from build123d import *

# Parameters (mm, degrees)
SKETCH1_R           = 22.86
BOSS_EXTRUDE1_DEPTH = 22.86
SKETCH3_R           = 15.24
BOSS_EXTRUDE2_DEPTH = 55.88
SKETCH4_R           = 22.86
BOSS_EXTRUDE3_DEPTH = 22.86
FILLET3_R           = 2.54
SKETCH5_R           = 2.055
CUT_EXTRUDE1_DEPTH  = 7.62
SKETCH8_W           = 3.7
SKETCH8_H           = 3.4
CUT_EXTRUDE2_DEPTH  = 85
FILLET4_R           = 1


with BuildPart() as part:
    # Sketch1 → Boss-Extrude1 (new body)
    with BuildSketch(Plane(origin=(0, 0, 0), x_dir=(1, 0, 0), z_dir=(0, 1, 0))):
        Circle(SKETCH1_R)
    extrude(amount=BOSS_EXTRUDE1_DEPTH)

    # Sketch3 → Boss-Extrude2 (add)
    with BuildSketch(Plane(origin=(0, 22.86, 0), x_dir=(1, 0, 0), z_dir=(0, 1, 0))):
        Circle(SKETCH3_R)
    extrude(amount=BOSS_EXTRUDE2_DEPTH)

    # Sketch4 → Boss-Extrude3 (add)
    with BuildSketch(Plane(origin=(0, 78.74, 0), x_dir=(1, 0, 0), z_dir=(0, 1, 0))):
        Circle(SKETCH4_R)
    extrude(amount=BOSS_EXTRUDE3_DEPTH)

    # Fillet3
    fillet3_edges = [part.edges().sort_by_distance(p)[0] for p in [
        (-22.86, 101.6, 0),
        (-22.86, 0, 0),
    ]]
    fillet(fillet3_edges, radius=FILLET3_R)

    # Sketch5 → Cut-Extrude1 (cut)
    with BuildSketch(Plane(origin=(0, 101.6, 0), x_dir=(1, 0, 0), z_dir=(0, 1, 0))):
        Circle(SKETCH5_R)
    extrude(amount=-CUT_EXTRUDE1_DEPTH, mode=Mode.SUBTRACT)

    # Sketch8 → Cut-Extrude2 (cut)
    with BuildSketch(Plane.XZ):
        Rectangle(SKETCH8_W, SKETCH8_H)
    extrude(amount=-CUT_EXTRUDE2_DEPTH, mode=Mode.SUBTRACT)

    # Fillet4
    fillet4_edges = [part.edges().sort_by_distance(p)[0] for p in [
        (-2.055, 101.6, 0),
        (-1.85, 0, 0),
        (0, 0, -1.7),
        (1.85, 0, 0),
        (0, 0, 1.7),
    ]]
    fillet(fillet4_edges, radius=FILLET4_R)


solid = part.part
Build history of the part. All positions in model axes, mm. A direction names the side the tool comes from. Round coordinates to 2 decimals unless told otherwise and drop trailing zeros. Write each loop counter-clockwise with the first axis right and the second up, starting at its lowest first coordinate (ties: lowest second). Pieces come first, ordered by that corner, then holes. Notation, with made-up numbers: M -37.75,-35.5 L -4.75,-35.5 A20 ccw -4.75,1.5 Z; hole C 30,73.5 d4. An arc over 180 degrees is marked long. Use CSV: the item, a comma, the result in double quotes.
1. Saw through at C-C (z = 0). Give the cut face in (x, y) (3 decimals), plus the area to 3 significant figures.
Reply:
outline,"M -22.86,2.54 A2.54 ccw -20.32,0 L -2.85,0 A1 ccw -1.85,1 L -1.85,85 L 1.85,85 L 1.85,1 A1 ccw 2.85,0 L 20.32,0 A2.54 ccw 22.86,2.54 L 22.86,22.86 L 15.24,22.86 L 15.24,78.74 L 22.86,78.74 L 22.86,99.06 A2.54 ccw 20.32,101.6 L 3.055,101.6 A1 ccw 2.055,100.6 L 2.055,93.98 L -2.055,93.98 L -2.055,100.6 A1 ccw -3.055,101.6 L -20.32,101.6 A2.54 ccw -22.86,99.06 L -22.86,78.74 L -15.24,78.74 L -15.24,22.86 L -22.86,22.86 Z"
area,"3,440 mm²"
2. Two-plate mould, pull along Z, no slides. Class faces 5 (the face through (0, 0, 4)), 6 (the face through (21.804, 88.758, -6.867)), 7 (the face through (0, 42, 1.7)): +Z half, -Z half, draft (parallel to the pull), parting line (faces both ways), or undercut.
Reply:
face 5,"draft"
face 6,"parting line"
face 7,"undercut"
3. Saw through at B-B (x = 0). Give the cut face in (y, z) (3 decimals), plus the area to 3 significant figures.
Reply:
outline,"M 0,-20.32 A2.54 ccw 2.54,-22.86 L 22.86,-22.86 L 22.86,-15.24 L 78.74,-15.24 L 78.74,-22.86 L 99.06,-22.86 A2.54 ccw 101.6,-20.32 L 101.6,-3.055 A1 ccw 100.6,-2.055 L 93.98,-2.055 L 93.98,2.055 L 100.6,2.055 A1 ccw 101.6,3.055 L 101.6,20.32 A2.54 ccw 99.06,22.86 L 78.74,22.86 L 78.74,15.24 L 22.86,15.24 L 22.86,22.86 L 2.54,22.86 A2.54 ccw 0,20.32 L 0,2.7 A1 ccw 1,1.7 L 85,1.7 L 85,-1.7 L 1,-1.7 A1 ccw 0,-2.7 Z"
area,"3,470 mm²"
4. Wall check: probe 1 along Y at (x, z) = (-5, 18.5); probe 2 along X at (y, z) = (96, 0) (3 decimals). Give the ranges that are in metal, low to high. Write a range as from..to.
Reply:
probe 1,"y = 0..22.86, 78.74..101.6"
probe 2,"x = -22.86..-2.055, 2.055..22.86"
5. Tool access for faces 1 (the face through (-1.85, 42, 0)), 2 (the face through (0, 101.6, 4)), 3 (the face through (-0.445, 97.336, 2.006)), 4 (the face through (5, 78.74, 15)): list every direction of +Z, -Z, +X, -X, +Y, -Y with a clear straight run to the whole face (end or side of a thin tool).
Reply:
face 1,"-Y"
face 2,"+Z, -Z, +X, -X, +Y"
face 3,"+Y"
face 4,"none"
6. Flat gauge pins, fed straight in: pin 1 (3.5 mm diameter, centred on y = 33, z = -0.5, fed in from +X); pin 2 (1.7 mm diameter, centred on x = -0.5, z = 0, fed in from -Y); pin 3 (3 mm diameter, centred on y = 78.5, z = 11, fed in from -X); pin 4 (5.5 mm diameter, centred on x = 0, z = 0, fed in from -Y). Where does each tip first touch, or does it go through?
Reply:
pin 1,"stops at x = 15.24"
pin 2,"stops at y = 85"
pin 3,"stops at x = -20.78"
pin 4,"stops at y = 0"
7. Saw through at D-D (y = 56). Give the cut face in (x, z).
Reply:
outline,"C 0,0 d30.48; hole M -1.85,-1.7 L 1.85,-1.7 L 1.85,1.7 L -1.85,1.7 Z"
8. Saw through at A-A (y = 13). Give the cut face in (x, z).
Reply:
outline,"C 0,0 d45.72; hole M -1.85,-1.7 L 1.85,-1.7 L 1.85,1.7 L -1.85,1.7 Z"
